```python
from build123d import *

# Parameters (mm, degrees)
SKETCH1_W                = 50
SKETCH1_H                = 50
BOSS_EXTRUDE1_DEPTH      = 2
BOSS_EXTRUDE2_DEPTH      = 1.2
BOSS_EXTRUDE2_DEPTH_BACK = 1.2
SKETCH3_W                = 1.1
SKETCH3_H                = 2.6
FILLET1_R                = 1
BOSS_EXTRUDE3_DEPTH      = 0.4
BOSS_EXTRUDE3_DEPTH_BACK = 1.2
SKETCH6_W                = 1.1
SKETCH6_H                = 4.6
FILLET2_R                = 0.3
FILLET3_R                = 0.3
CUT_EXTRUDE1_REACH       = 38.287
SKETCH7_R                = 5
FILLET5_R                = 1


# Some blends are built 0.0001 mm under size
with BuildPart() as part:
    # Sketch1 → Boss-Extrude1 (new body)
    with BuildSketch(Plane.XY):
        Rectangle(SKETCH1_W, SKETCH1_H)
    extrude(amount=BOSS_EXTRUDE1_DEPTH)

    # Sketch3 → Boss-Extrude2 (add, two sides: drawn at the far end of the back side and taken through both)
    with BuildSketch(Plane.ZY.offset(25).offset(-BOSS_EXTRUDE2_DEPTH_BACK)):
        with Locations((0.25, 19.8)):
            Rectangle(SKETCH3_W, SKETCH3_H)
        with Locations((0.25, -19.8)):
            Rectangle(SKETCH3_W, SKETCH3_H)
    extrude(amount=BOSS_EXTRUDE2_DEPTH + BOSS_EXTRUDE2_DEPTH_BACK)

    # Fillet1
    # the kernel refuses this fillet: 1 mm, written as the material it adds along each edge
    with BuildSketch(Plane(origin=(-23.8, 21.1, 0), x_dir=(0, 1, 0), z_dir=(-1, 0, 0)), Plane(origin=(-25, 18.5, 0), x_dir=(0, -1, 0), z_dir=(1, 0, 0))) as fillet1_piece_1:
        with BuildLine():
            CenterArc((0.714142843, 1), FILLET1_R, 224.427004001, 45.572995999)
            Line((0, 0.3), (-0.014282857, 0.286))
            ThreePointArc((-0.014282857, 0.286), (-0.02, 0.15), (-0.02, 0))
            Line((-0.02, 0), (0, -0.02))
            Line((0, -0.02), (0.714142843, -0.02))
            Line((0.714142843, -0.02), (0.714142843, 0))
        make_face()
    extrude(amount=1.2)
    with BuildSketch(Plane(origin=(-23.8, -21.1, 0), x_dir=(0, -1, 0), z_dir=(-1, 0, 0)), Plane(origin=(-25, -18.5, 0), x_dir=(0, 1, 0), z_dir=(1, 0, 0))) as fillet1_piece_2:
        with BuildLine():
            CenterArc((0.714142843, -1), FILLET1_R, 90, 45.572995999)
            Line((0, -0.3), (-0.014282857, -0.286))
            ThreePointArc((-0.014282857, -0.286), (-0.02, -0.15), (-0.02, 0))
            Line((-0.02, 0), (0, 0.02))
            Line((0, 0.02), (0.714142843, 0.02))
            Line((0.714142843, 0.02), (0.714142843, 0))
        make_face()
    extrude(amount=1.2)
    with BuildSketch(Plane(origin=(-23.8, -18.5, 0), x_dir=(1, 0, 0), z_dir=(0, -1, 0))) as fillet1_piece_3:
        with BuildLine():
            CenterArc((0.714142843, -1), FILLET1_R, 90, 45.572995999)
            Line((0, -0.3), (-0.014282857, -0.286))
            ThreePointArc((-0.014282857, -0.286), (-0.02, -0.15), (-0.02, 0))
            Line((-0.02, 0), (0, 0.02))
            Line((0, 0.02), (0.714142843, 0.02))
            Line((0.714142843, 0.02), (0.714142843, 0))
        make_face()
    extrude(amount=2.6)
    with BuildSketch(Plane(origin=(-23.8, 18.5, 0), x_dir=(1, 0, 0), z_dir=(0, 1, 0))) as fillet1_piece_4:
        with BuildLine():
            CenterArc((0.714142843, 1), FILLET1_R, 224.427004001, 45.572995999)
            Line((0, 0.3), (-0.014282857, 0.286))
            ThreePointArc((-0.014282857, 0.286), (-0.02, 0.15), (-0.02, 0))
            Line((-0.02, 0), (0, -0.02))
            Line((0, -0.02), (0.714142843, -0.02))
            Line((0.714142843, -0.02), (0.714142843, 0))
        make_face()
    extrude(amount=2.6)
    with BuildSketch(Plane(origin=(-25, -21.1, 0.8), x_dir=(0, 0, 1), z_dir=(0, 1, 0))) as fillet1_piece_5:
        with BuildLine():
            CenterArc((FILLET1_R, -FILLET1_R), FILLET1_R, 90, 90)
            Line((0, -FILLET1_R), (-FILLET1_R * 0.02, -FILLET1_R))
            Line((-FILLET1_R * 0.02, -FILLET1_R), (-FILLET1_R * 0.02, FILLET1_R * 0.02))
            Line((-FILLET1_R * 0.02, FILLET1_R * 0.02), (FILLET1_R, FILLET1_R * 0.02))
            Line((FILLET1_R, FILLET1_R * 0.02), (FILLET1_R, 0))
        make_face()
    extrude(amount=2.6)
    with BuildSketch(Plane(origin=(-25, 21.1, 0.8), x_dir=(0, 0, 1), z_dir=(0, -1, 0))) as fillet1_piece_6:
        with BuildLine():
            CenterArc((FILLET1_R, FILLET1_R), FILLET1_R, 180, 90)
            Line((0, FILLET1_R), (-FILLET1_R * 0.02, FILLET1_R))
            Line((-FILLET1_R * 0.02, FILLET1_R), (-FILLET1_R * 0.02, -FILLET1_R * 0.02))
            Line((-FILLET1_R * 0.02, -FILLET1_R * 0.02), (FILLET1_R, -FILLET1_R * 0.02))
            Line((FILLET1_R, -FILLET1_R * 0.02), (FILLET1_R, 0))
        make_face()
    extrude(amount=2.6)
    with BuildSketch(Plane(origin=(-22.014642893, 21.1, 0), x_dir=(0, 1, 0), z_dir=(-1, 0, 0))) as fillet1_piece_7a_section:
        with BuildLine():
            CenterArc((0.714142843, 1), FILLET1_R, 224.427004001, 45.572995999)
            Line((0, 0.3), (-0.014282857, 0.286))
            ThreePointArc((-0.014282857, 0.286), (-0.02, 0.15), (-0.02, 0))
            Line((-0.02, 0), (0, -0.02))
            Line((0, -0.02), (0.714142843, -0.02))
            Line((0.714142843, -0.02), (0.714142843, 0))
        make_face()
    fillet1_piece_7a = extrude(amount=2.985357107, mode=Mode.PRIVATE)
    fillet1_piece_7a = split(fillet1_piece_7a, bisect_by=Plane(origin=(-23.8, 21.290996304, -0.074177971), z_dir=(1, 0, 0)), keep=Keep.TOP, mode=Mode.PRIVATE)
    with BuildSketch(Plane(origin=(-23.8, 18.5, 0), x_dir=(1, 0, 0), z_dir=(0, 1, 0))) as fillet1_piece_7b_section:
        with BuildLine():
            CenterArc((0.714142843, 1), FILLET1_R, 224.427004001, 45.572995999)
            Line((0, 0.3), (-0.014282857, 0.286))
            ThreePointArc((-0.014282857, 0.286), (-0.02, 0.15), (-0.02, 0))
            Line((-0.02, 0), (0, -0.02))
            Line((0, -0.02), (0.714142843, -0.02))
            Line((0.714142843, -0.02), (0.714142843, 0))
        make_face()
    fillet1_piece_7b = extrude(amount=4.385357107, mode=Mode.PRIVATE)
    fillet1_piece_7b = split(fillet1_piece_7b, bisect_by=Plane(origin=(-23.609003696, 21.1, -0.074177971), z_dir=(0, 1, 0)), keep=Keep.TOP, mode=Mode.PRIVATE)
    fillet1_piece_7 = fillet1_piece_7a & fillet1_piece_7b
    add(fillet1_piece_7)
    with BuildSketch(Plane(origin=(-23.8, 16.714642893, 0), x_dir=(1, 0, 0), z_dir=(0, 1, 0))) as fillet1_piece_8a_section:
        with BuildLine():
            CenterArc((0.714142843, 1), FILLET1_R, 224.427004001, 45.572995999)
            Line((0, 0.3), (-0.014282857, 0.286))
            ThreePointArc((-0.014282857, 0.286), (-0.02, 0.15), (-0.02, 0))
            Line((-0.02, 0), (0, -0.02))
            Line((0, -0.02), (0.714142843, -0.02))
            Line((0.714142843, -0.02), (0.714142843, 0))
        make_face()
    fillet1_piece_8a = extrude(amount=4.385357107, mode=Mode.PRIVATE)
    fillet1_piece_8a = split(fillet1_piece_8a, bisect_by=Plane(origin=(-23.609003696, 18.5, -0.074177971), z_dir=(0, -1, 0)), keep=Keep.TOP, mode=Mode.PRIVATE)
    with BuildSketch(Plane(origin=(-25, 18.5, 0), x_dir=(0, -1, 0), z_dir=(1, 0, 0))) as fillet1_piece_8b_section:
        with BuildLine():
            CenterArc((0.714142843, 1), FILLET1_R, 224.427004001, 45.572995999)
            Line((0, 0.3), (-0.014282857, 0.286))
            ThreePointArc((-0.014282857, 0.286), (-0.02, 0.15), (-0.02, 0))
            Line((-0.02, 0), (0, -0.02))
            Line((0, -0.02), (0.714142843, -0.02))
            Line((0.714142843, -0.02), (0.714142843, 0))
        make_face()
    fillet1_piece_8b = extrude(amount=2.985357107, mode=Mode.PRIVATE)
    fillet1_piece_8b = split(fillet1_piece_8b, bisect_by=Plane(origin=(-23.8, 18.309003696, -0.074177971), z_dir=(1, 0, 0)), keep=Keep.TOP, mode=Mode.PRIVATE)
    fillet1_piece_8 = fillet1_piece_8a & fillet1_piece_8b
    add(fillet1_piece_8)
    with BuildSketch(Plane(origin=(-23.8, -18.5, 0), x_dir=(1, 0, 0), z_dir=(0, -1, 0))) as fillet1_piece_9a_section:
        with BuildLine():
            CenterArc((0.714142843, -1), FILLET1_R, 90, 45.572995999)
            Line((0, -0.3), (-0.014282857, -0.286))
            ThreePointArc((-0.014282857, -0.286), (-0.02, -0.15), (-0.02, 0))
            Line((-0.02, 0), (0, 0.02))
            Line((0, 0.02), (0.714142843, 0.02))
            Line((0.714142843, 0.02), (0.714142843, 0))
        make_face()
    fillet1_piece_9a = extrude(amount=4.385357107, mode=Mode.PRIVATE)
    fillet1_piece_9a = split(fillet1_piece_9a, bisect_by=Plane(origin=(-23.609003696, -21.1, -0.074177971), z_dir=(0, -1, 0)), keep=Keep.TOP, mode=Mode.PRIVATE)
    with BuildSketch(Plane(origin=(-22.014642893, -21.1, 0), x_dir=(0, -1, 0), z_dir=(-1, 0, 0))) as fillet1_piece_9b_section:
        with BuildLine():
            CenterArc((0.714142843, -1), FILLET1_R, 90, 45.572995999)
            Line((0, -0.3), (-0.014282857, -0.286))
            ThreePointArc((-0.014282857, -0.286), (-0.02, -0.15), (-0.02, 0))
            Line((-0.02, 0), (0, 0.02))
            Line((0, 0.02), (0.714142843, 0.02))
            Line((0.714142843, 0.02), (0.714142843, 0))
        make_face()
    fillet1_piece_9b = extrude(amount=2.985357107, mode=Mode.PRIVATE)
    fillet1_piece_9b = split(fillet1_piece_9b, bisect_by=Plane(origin=(-23.8, -21.290996304, -0.074177971), z_dir=(1, 0, 0)), keep=Keep.TOP, mode=Mode.PRIVATE)
    fillet1_piece_9 = fillet1_piece_9a & fillet1_piece_9b
    add(fillet1_piece_9)
    with BuildSketch(Plane(origin=(-25, -18.5, 0), x_dir=(0, 1, 0), z_dir=(1, 0, 0))) as fillet1_piece_10a_section:
        with BuildLine():
            CenterArc((0.714142843, -1), FILLET1_R, 90, 45.572995999)
            Line((0, -0.3), (-0.014282857, -0.286))
            ThreePointArc((-0.014282857, -0.286), (-0.02, -0.15), (-0.02, 0))
            Line((-0.02, 0), (0, 0.02))
            Line((0, 0.02), (0.714142843, 0.02))
            Line((0.714142843, 0.02), (0.714142843, 0))
        make_face()
    fillet1_piece_10a = extrude(amount=2.985357107, mode=Mode.PRIVATE)
    fillet1_piece_10a = split(fillet1_piece_10a, bisect_by=Plane(origin=(-23.8, -18.309003696, -0.074177971), z_dir=(1, 0, 0)), keep=Keep.TOP, mode=Mode.PRIVATE)
    with BuildSketch(Plane(origin=(-23.8, -16.714642893, 0), x_dir=(1, 0, 0), z_dir=(0, -1, 0))) as fillet1_piece_10b_section:
        with BuildLine():
            CenterArc((0.714142843, -1), FILLET1_R, 90, 45.572995999)
            Line((0, -0.3), (-0.014282857, -0.286))
            ThreePointArc((-0.014282857, -0.286), (-0.02, -0.15), (-0.02, 0))
            Line((-0.02, 0), (0, 0.02))
            Line((0, 0.02), (0.714142843, 0.02))
            Line((0.714142843, 0.02), (0.714142843, 0))
        make_face()
    fillet1_piece_10b = extrude(amount=4.385357107, mode=Mode.PRIVATE)
    fillet1_piece_10b = split(fillet1_piece_10b, bisect_by=Plane(origin=(-23.609003696, -18.5, -0.074177971), z_dir=(0, 1, 0)), keep=Keep.TOP, mode=Mode.PRIVATE)
    fillet1_piece_10 = fillet1_piece_10a & fillet1_piece_10b
    add(fillet1_piece_10)

    # Sketch6 → Boss-Extrude3 (add, two sides: drawn at the far end of the back side and taken through both)
    with BuildSketch(Plane(origin=(25, 0, 0), x_dir=(0, 0, -1), z_dir=(1, 0, 0)).offset(-BOSS_EXTRUDE3_DEPTH_BACK)):
        with Locations((-0.25, 0)):
            Rectangle(SKETCH6_W, SKETCH6_H)
    extrude(amount=BOSS_EXTRUDE3_DEPTH + BOSS_EXTRUDE3_DEPTH_BACK)

    # Fillet2
    fillet2_edges = [part.edges().sort_by_distance(p)[0] for p in [
        (25.4, 2.3, 0.25),
        (25.4, -2.3, 0.25),
        (25.4, 0, 0.8),
        (25.4, 0, -0.3),
    ]]
    fillet(fillet2_edges, radius=FILLET2_R)

    # Fillet3
    fillet3_edges = [part.edges().sort_by_distance(p)[0] for p in [
        (24.4, -2.3, 0),
        (24.4, 2.3, 0),
        (23.8, 0, 0),
    ]]
    fillet(fillet3_edges, radius=FILLET3_R - 0.0001)  # a hair under: the kernel refuses the full size

    # Sketch7 → Cut-Extrude1 (cut, up to next)
    with BuildSketch(Plane.XY.offset(2), mode=Mode.PRIVATE) as cut_extrude1_sk1:
        with Locations((15, 0)):
            Circle(SKETCH7_R)
    cut_extrude1_tool1 = extrude(cut_extrude1_sk1.sketch, amount=-CUT_EXTRUDE1_REACH, mode=Mode.PRIVATE) & part.part
    add(cut_extrude1_tool1.solids().sort_by_distance((15, 0, 2))[0], mode=Mode.SUBTRACT)

    # Fillet5
    fillet5_edges = [part.edges().sort_by_distance(p)[0] for p in [
        (10, 0, 2),
        (10, 0, 0),
    ]]
    fillet(fillet5_edges, radius=FILLET5_R - 0.0001)  # a hair under: the kernel refuses the full size


solid = part.part
```
Here's how the part is built. I have some questions about the finished solid (model axes, mm). A direction names the side the tool comes from. Round coordinates to 2 decimals unless told otherwise and drop trailing zeros. Loops run counter-clockwise (first coordinate to the right, second up) from the corner with the lowest first, then second, coordinate; pieces in that order, holes last.
1. Will these pins go through, and if not, where does the flat tip stop? pin 1 (4 mm diameter, centred on x = -16.5, y = 10.5, fed in from -Z); pin 2 (8 mm diameter, centred on x = 15, y = 0, fed in from -Z).
Answers:
pin 1: stops at z = 0
pin 2: passes through
2. Thinking about a two-plate mould opening in Y: for faces 1 (the face through (-25, 20, -0.3)), 2 (the face through (-25, 0, 1)), 3 (the face through (-26, 18.5, 0)), 4 (the face through (-26, -21.1, 0)), which applies, released by +Y, released by -Y, zero draft, split by the parting line, or undercut?
Answers:
face 1: zero draft
face 2: undercut
face 3: undercut
face 4: released by -Y
3. For faces 5 (the face through (-26, 21.1, 0)), 6 (the face through (-26, -18.5, 0)), 7 (the face through (24, 0, -0.3)), which set-ups out of +Z, -Z, +X, -X, +Y, -Y let a thin tool reach every point of the face, with its end or its side?
Answers:
face 5: +Z, -Z, -X, +Y
face 6: +Z, -Z, -X
face 7: -Z, +X, -X, +Y, -Y
4. If I drill on probe 1 along Y at (x, z) = (15, 1); probe 2 along X at (y, z) = (17, 0.55); probe 3 along Z at (x, y) = (-12.5, 11), over which ranges is the centre line in solid material (lowest first)?
Answers:
probe 1: y = -25 to -5, 5 to 25
probe 2: x = -25 to 25
probe 3: z = 0 to 2
5. Suppose I cut it at C-C, the plane y = -11. Please give me the cut outline in (x, z), and give its area (3 significant figures).
Answers:
outline: (-25, 0) - (25, 0) - (25, 2) - (-25, 2) - close
area: 100 mm2
